Here's how the part is built. I have some questions about the finished solid (model axes, mm). Give positions to 0.01 mm unless a question says otherwise; leave off trailing zeros. Loops run counter-clockwise (first coordinate to the right, second up) from the corner with the lowest first, then second, coordinate; pieces in that order, holes last.
Q1. Suppose I cut it at B-B (y = 29). List the corners of the cut face in (x, z) for me.
Q2. I'm going to push flat-ended pins straight in: P1, Ø6, axis at x = -15, z = -437.5, coming from the -Y side; P2, Ø11.5, axis at x = -15, z = -237.5, coming from the +Y side; P3, Ø12.5, axis at y = 34, z = -453.5, coming from the -X side. Where does each tip first touch, or does it pass through?
Q3. I need wall thicknesses on probe 1 along Z at (x, y) = (-15, 0.7); probe 2 along X at (y, z) = (42, -156.5); probe 3 along Y at (x, z) = (-22.5, -101). Which ranges of each line are inside material? Lowest first, please.
Q4. Suppose I cut it at A-A (z = -300.5). List the corners of the cut face in (x, y) for me.
```python
from build123d import *

# Parameters (mm, degrees)
SKETCH1_W                    = 675
SKETCH1_H                    = 45
BASE_FLANGE1_DEPTH           = 2.5
EDGE_FLANGE1_STRIP_W         = 11.4732
EDGE_FLANGE1_STRIP_H         = 2.5
EDGE_FLANGE1_STRIP_CUT_DEPTH = 675
EDGE_FLANGE1_DEPTH           = 675
SKETCH9_R                    = 5
CUT_EXTRUDE1_DEPTH           = 10
LPATTERN1_COUNT              = 4
LPATTERN1_PITCH              = 200


# Sheet-metal steps are written as plain solids
with BuildPart() as part:
    # Sketch1 → Base-Flange1 (new body)
    with BuildSketch(Plane(origin=(0, 0, 0), x_dir=(0, 0, -1), z_dir=(1, 0, 0))):
        with Locations((337.5, 22.5)):
            Rectangle(SKETCH1_W, SKETCH1_H)
    extrude(amount=-BASE_FLANGE1_DEPTH)

    # Edge-Flange1 strip (across the edge) → Edge-Flange1 strip cut (cut)
    with BuildSketch(Plane(origin=(-2.5, 0, -675), x_dir=(0, 1, 0), z_dir=(0, 0, 1))):
        with Locations((-2.5, -1.25)):
            Rectangle(EDGE_FLANGE1_STRIP_W, EDGE_FLANGE1_STRIP_H)
    extrude(amount=EDGE_FLANGE1_STRIP_CUT_DEPTH, mode=Mode.SUBTRACT)

    # Edge-Flange1 section (across the edge) → Edge-Flange1 (add)
    with BuildSketch(Plane(origin=(-2.5, 0, -675), x_dir=(0, 1, 0), z_dir=(0, 0, 1))):
        with BuildLine():
            Line((0, 0.7366), (0, 27.5))
            Line((0, 27.5), (2.5, 27.5))
            Line((2.5, 27.5), (2.5, 0.7366))
            ThreePointArc((2.5, 0.7366), (2.715745145, 0.215745145), (3.2366, 0))
            Line((3.2366, 0), (3.2366, -2.5))
            ThreePointArc((3.2366, -2.5), (0.947978192, -1.552021808), (0, 0.7366))
        make_face()
    extrude(amount=EDGE_FLANGE1_DEPTH)

    # Sketch9 → Cut-Extrude1 (cut)
    with BuildSketch(Plane(origin=(0, 0, 0), x_dir=(-1, 0, 0), z_dir=(0, -1, 0))):
        with Locations(Location((15, 637.5, 0), (0, 0, 180))):
            Circle(SKETCH9_R)
    cut_extrude1 = extrude(amount=-CUT_EXTRUDE1_DEPTH, mode=Mode.SUBTRACT)

    # LPattern1: Cut-Extrude1 ×4
    with Locations(*[(0, 0, i * LPATTERN1_PITCH) for i in range(1, LPATTERN1_COUNT)]):
        add(cut_extrude1, mode=Mode.SUBTRACT)


solid = part.part
```
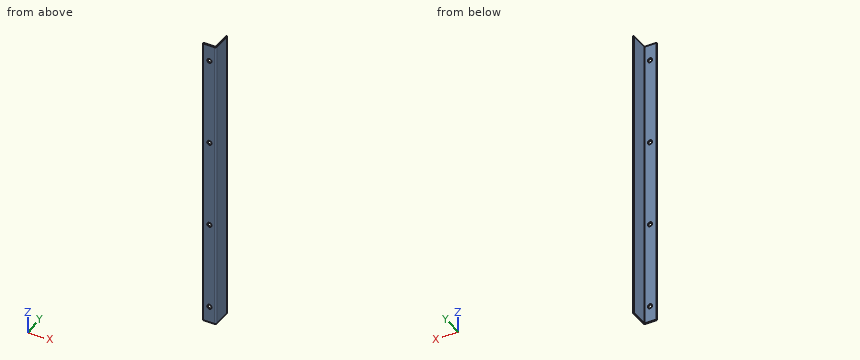
Solutions:
1. outline: (-2.5, -675) - (0, -675) - (0, 0) - (-2.5, 0) - close
2. P1: passes through
2. P2: stops at y = 2.5
2. P3: stops at x = -2.5
3. probe 1: z = -675 to -642.5, -632.5 to -442.5, -432.5 to -242.5, -232.5 to -42.5, -32.5 to 0
3. probe 2: x = -2.5 to 0
3. probe 3: y = 0 to 2.5
4. outline: (-30, 0) - (-3.24, 0) arc R3.24 ccw to (0, 3.24) - (0, 45) - (-2.5, 45) - (-2.5, 3.24) arc R0.74 cw to (-3.24, 2.5) - (-30, 2.5) - close
